Design review of the part shown in the three views and the two pictorial views. Dimensions are in mm from the part's minimum x, y and z. A direction names the side the tool comes from. Round coordinates to 2 decimals unless told otherwise and drop trailing zeros. Order: outer loops, then holes, each group sorted by start corner. A loop starts at its lowest first (then second) coordinate and runs counter-clockwise, first axis right, second up.
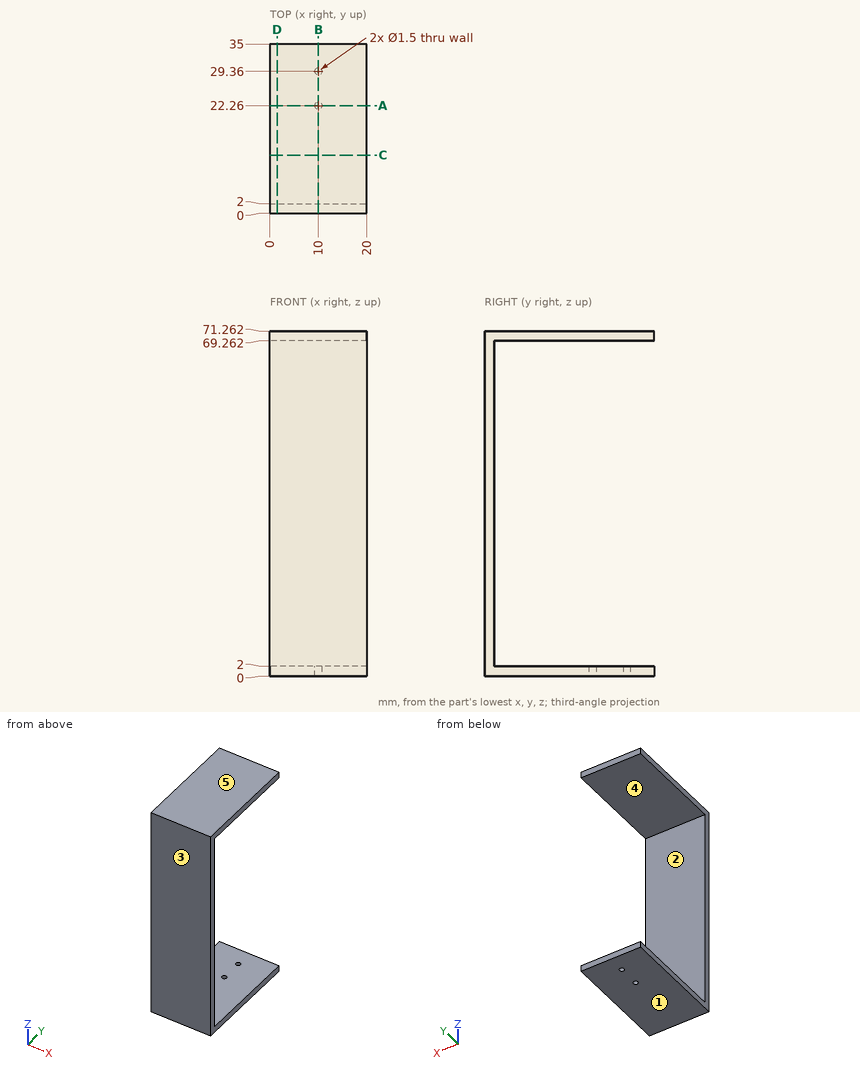
(1) Draft analysis for pull direction Z (two halves, no side actions). For the marked faces 1, 2 and 3, state which applies: pulls with the +Z half, pulls with the -Z half, needs draft (parallel to the pull), parting line crosses it, or undercut.
Data:
face 1: pulls with the -Z half
face 2: undercut
face 3: needs draft
(2) For the marked faces 4 and 5, list the 3-axis set-ups (+Z, -Z, +X, -X, +Y, -Y) from which the entire face can be reached by the end or side of a thin tool; tool diameter is ignored.
Data:
face 4: +X, -X, +Y
face 5: +Z, +X, -X, +Y, -Y
(3) Consider section D-D (x = 1.5). Write out the cut boundary in (y, z).
Data:
outline: (0, 0) - (35, 0) - (35, 2) - (2, 2) - (2, 69.26) - (35, 69.26) - (35, 71.26) - (0, 71.26) - close
(4) Consider section A-A (y = 22.26). Write out the cut boundary in (x, z), and give its area (3 significant figures).
Data:
outline: (0, 0) - (9.25, 0) - (9.25, 2) - (0, 2) - close; (0, 69.26) - (20, 69.26) - (20, 71.26) - (0, 71.26) - close; (10.75, 0) - (20, 0) - (20, 2) - (10.75, 2) - close
area: 77.0 mm2
(5) Consider section B-B (x = 10). Write out the cut boundary in (y, z).
Data:
outline: (0, 0) - (21.51, 0) - (21.51, 2) - (2, 2) - (2, 69.26) - (35, 69.26) - (35, 71.26) - (0, 71.26) - close; (23.01, 0) - (28.61, 0) - (28.61, 2) - (23.01, 2) - close; (30.11, 0) - (35, 0) - (35, 2) - (30.11, 2) - close
(6) Consider section C-C (y = 12). Write out the cut boundary in (x, z), and give its area (3 significant figures).
Data:
outline: (0, 0) - (20, 0) - (20, 2) - (0, 2) - close; (0, 69.26) - (20, 69.26) - (20, 71.26) - (0, 71.26) - close
area: 80.0 mm2
(7) To check wall thickness, follow probe 1 along Y at (x, z) = (10, 1.25); probe 2 along Z at (x, y) = (5, 22); probe 3 along Y at (x, z) = (15, 44). State the ranges of each line that lie inside material, in increasing order.
Data:
probe 1: y = 0 to 21.51, 23.01 to 28.61, 30.11 to 35
probe 2: z = 0 to 2, 69.26 to 71.26
probe 3: y = 0 to 2
(8) Insertion check: pin 1 (12 mm diameter, centred on x = 4, z = 44.5, fed in from +Y). The pin has a flat end and moves straight along its axis. Give the tip position at first contact, or say it passes through.
Data:
pin 1: stops at y = 2
